from build123d import *

# Parameters (mm, degrees)
SKETCH1_R            = 40
BOSS_EXTRUDE1_DEPTH  = 1.5875
M4_CLEARANCE_HOLE1_D = 4.5


with BuildPart() as part:
    # Sketch1 → Boss-Extrude1 (new body, symmetric)
    with BuildSketch(Plane.XY):
        Circle(SKETCH1_R)
    extrude(amount=BOSS_EXTRUDE1_DEPTH, both=True)

    # M4 Clearance Hole1 (through all)
    with Locations(Plane(origin=(0, 0, -1.5875), x_dir=(-1, 0, 0), z_dir=(0, 0, -1))):
        with Locations((15, 19.125), (-15, 19.125), (-15, -19.125), (15, -19.125)):
            Hole(M4_CLEARANCE_HOLE1_D / 2)


solid = part.part
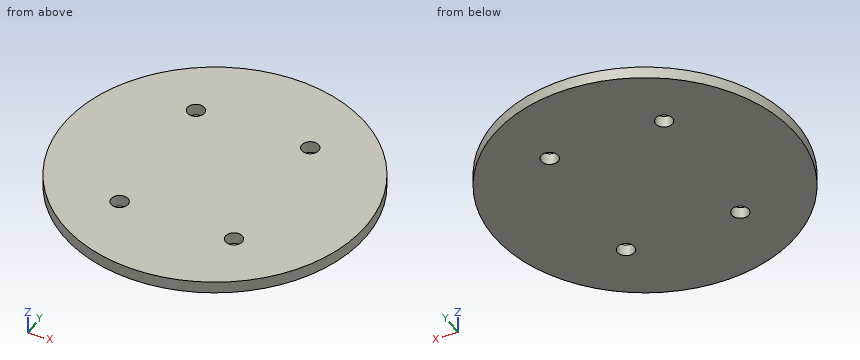
Model file for the job. Use its own axes, mm. Give positions to 0.01 mm unless a question says otherwise; leave off trailing zeros. Order: outer loops, then holes, each group sorted by start corner. A loop starts at its lowest first (then second) coordinate and runs counter-clockwise, first axis right, second up. Notation, with made-up numbers: M 24.25,53.25 L 45.25,53.25 A19 ccw 45.25,69.25 Z; hole C 20.5,85.25 d2. An arc over 180 degrees is marked long. Put each result on its own line as item: value. Start each with the question number.
(1) Band-saw the part on A-A on x = -15. Give the cut face in (y, z) (1 decimal).
(2) Band-saw the part on D-D on x = -25. Give the cut face in (y, z), then the cut area to 3 significant figures.
(3) Drill centre lines: L1, parallel to Y at x = -15, z = 0.1 (3 decimals); L2, parallel to Y at x = -13.5, z = -1.1; L3, parallel to X at y = 33.5, z = 1. Where is each one in solid material? Low to high. Write a range as [from, to].
(4) Pin check, flat tips, straight feed: pin 1 Ø1.5 at (y, z) = (-4.5, 0.5) entering from -X; pin 2 Ø1.5 at (x, z) = (-25.5, -1) entering from +Y; pin 3 Ø1.5 at (x, z) = (25.5, -0.5) entering from -Y. Stop position of each tip, or through.
(5) Band-saw the part on C-C on y = -34. Give the cut face in (x, z).
(6) Band-saw the part on B-B on z = 0.2. Give the cut face in (x, y) (3 decimals).
Results below:
1. outline: M -37.1,-1.6 L -21.4,-1.6 L -21.4,1.6 L -37.1,1.6 Z; M -16.9,-1.6 L 16.9,-1.6 L 16.9,1.6 L -16.9,1.6 Z; M 21.4,-1.6 L 37.1,-1.6 L 37.1,1.6 L 21.4,1.6 Z
2. outline: M -31.22,-1.59 L 31.22,-1.59 L 31.22,1.59 L -31.22,1.59 Z
2. area: 198 mm2
3. L1: y = [-37.081, -21.375], [-16.875, 16.875], [21.375, 37.081]
3. L2: y = [-37.65, -20.8], [-17.45, 17.45], [20.8, 37.65]
3. L3: x = [-21.86, 21.86]
4. pin 1: stops at x = -39.82
4. pin 2: stops at y = 31.42
4. pin 3: stops at y = -31.42
5. outline: M -21.07,-1.59 L 21.07,-1.59 L 21.07,1.59 L -21.07,1.59 Z
6. outline: C 0,0 d80; hole C -15,-19.125 d4.5; hole C -15,19.125 d4.5; hole C 15,-19.125 d4.5; hole C 15,19.125 d4.5
